For this review, take the finished solid that the model builds, in its own axes (mm). A direction names the side the tool comes from. Give positions to 0.01 mm unless a question says otherwise; leave off trailing zeros. Loops run counter-clockwise (first coordinate to the right, second up) from the corner with the lowest first, then second, coordinate; pieces in that order, holes last. Notation, with made-up numbers: (67, 11) - (94, 11) arc R14 ccw to (94, 35) - close; hole circle Ø8 at (31, -13). An arc over 180 degrees is marked (long way). Answer as CSV lines item,"result".
from build123d import *

# Parameters (mm, degrees)
BASE_FLANGE1_DEPTH = 111.125
SKETCH16_R         = 14.2875
SKETCH16_R_2       = 2.5146
CUT_EXTRUDE1_DEPTH = 191.975656171


# Read off the part's stored shape, not the designer's step: Base-Flange1
with BuildPart() as part:
    # Base-Flange1 outline → Base-Flange1 (new body)
    with BuildSketch(Plane.XY):
        with BuildLine():
            Line((98.425, -3.937), (98.425, -117.475))
            Line((98.425, -117.475), (101.6, -117.475))
            Line((101.6, -117.475), (101.6, -3.937))
            ThreePointArc((101.6, -3.937), (100.446879398, -1.153120602), (97.663, 0))
            Line((97.663, 0), (0, 0))
            Line((0, 0), (0, -3.175))
            Line((0, -3.175), (97.663, -3.175))
            ThreePointArc((97.663, -3.175), (98.201815367, -3.398184633), (98.425, -3.937))
        make_face()
    extrude(amount=BASE_FLANGE1_DEPTH)

    # Sketch16 → Cut-Extrude1 (cut, through all)
    with BuildSketch(Plane(origin=(101.6, 0, 0), x_dir=(0, 0, -1), z_dir=(1, 0, 0))):
        with Locations((-31.75, -84.1375)):
            Circle(SKETCH16_R)
        with Locations((-95.25, -39.6875)):
            Circle(SKETCH16_R)
        with Locations((-38.1, -15.875)):
            Circle(SKETCH16_R_2)
        with Locations((-38.1, -34.925)):
            Circle(SKETCH16_R_2)
        with Locations((-57.15, -15.875)):
            Circle(SKETCH16_R_2)
        with Locations((-57.15, -34.925)):
            Circle(SKETCH16_R_2)
        with Locations((-19.05, -15.875)):
            Circle(SKETCH16_R_2)
        with Locations((-19.05, -34.925)):
            Circle(SKETCH16_R_2)
        Polygon((-58.7375, -117.475), (-111.125, -44.592589994), (-111.125, -117.475), align=None)
    extrude(amount=-CUT_EXTRUDE1_DEPTH, mode=Mode.SUBTRACT)


solid = part.part
1) Wall thickness on line 1 (Y direction, x = 100.35, z = 57.15) (1 decimal); line 2 (X direction, y = -36.5, z = 79.5) (3 decimals); line 3 (Y direction, x = 24, z = 9) (3 decimals): over which ranges is each line inside the solid? List them lowest first. Write a range as from..to.
From the geometry:
line 1,"y = -117.5..-37.4, -32.4..-18.4, -13.4..-1.1"
line 2,"x = 98.425..101.6"
line 3,"y = -3.175..0"
2) Consider section A-A on z = 57.15. Write out the cut boundary in (x, y) (3 decimals), and give its area (3 significant figures).
From the geometry:
outline,"(0, -3.175) - (97.663, -3.175) arc R0.762 cw to (98.425, -3.937) - (98.425, -13.36) - (101.6, -13.36) - (101.6, -3.937) arc R3.937 ccw to (97.663, 0) - (0, 0) - close; (98.425, -117.475) - (101.6, -117.475) - (101.6, -37.44) - (98.425, -37.44) - close; (98.425, -32.41) - (101.6, -32.41) - (101.6, -18.39) - (98.425, -18.39) - close"
area,"650 mm^2"
3) Consider section D-D on z = 38.1. Write out the cut boundary in (x, y) (3 decimals).
From the geometry:
outline,"(0, -3.175) - (97.663, -3.175) arc R0.762 cw to (98.425, -3.937) - (98.425, -13.36) - (101.6, -13.36) - (101.6, -3.937) arc R3.937 ccw to (97.663, 0) - (0, 0) - close; (98.425, -117.475) - (101.6, -117.475) - (101.6, -96.936) - (98.425, -96.936) - close; (98.425, -71.339) - (101.6, -71.339) - (101.6, -37.44) - (98.425, -37.44) - close; (98.425, -32.41) - (101.6, -32.41) - (101.6, -18.39) - (98.425, -18.39) - close"
4) Insertion check: P1, Ø6, axis at y = -15.875, z = 57.15, coming from the -X side (3 decimals); P2, Ø8, axis at x = 46.5, z = 17, coming from the -Y side (3 decimals). Each pin has a flat end and moves straight along its axis. Give the tip position at first contact, or say it passes through.
From the geometry:
P1,"stops at x = 98.425"
P2,"stops at y = -3.175"
5) Consider section B-B on y = -49.5. Write out the cut boundary in (x, z) (3 decimals), and give its area (3 significant figures).
From the geometry:
outline,"(98.425, 0) - (101.6, 0) - (101.6, 84.865) - (98.425, 84.865) - close; (98.425, 105.635) - (101.6, 105.635) - (101.6, 107.598) - (98.425, 107.598) - close"
area,"276 mm^2"
6) Machinability: for faces 1 (the cylindrical face through (100.035, -33.226, 20.903)), 2 (the flat face through (98.425, -47, 42)), which of the approach directions +Z, -Z, +X, -X, +Y, -Y give a long, thin tool a straight path to every point of the face, cutting with its end or side? Answer none if there is none.
From the geometry:
face 1,"+X, -X"
face 2,"+Z, -Z, -X, -Y"
7) Draft analysis for pull direction Z (two halves, no side actions). For faces 3 (the cylindrical face through (100.03, -34.17, 54.75)), 4 (the flat face through (66, -2, 111.125)), 5 (the cylindrical face through (100.03, -15.12, 54.75)), 6 (the flat face through (101.6, -49, 42)), state which applies: pulls with the +Z half, pulls with the -Z half, needs draft (parallel to the pull), parting line crosses it, or undercut.
From the geometry:
face 3,"undercut"
face 4,"pulls with the +Z half"
face 5,"undercut"
face 6,"needs draft"
8) Consider section C-C on z = 95.25. Write out the cut boundary in (x, y) (3 decimals), and give its area (3 significant figures).
From the geometry:
outline,"(0, -3.175) - (97.663, -3.175) arc R0.762 cw to (98.425, -3.937) - (98.425, -25.4) - (101.6, -25.4) - (101.6, -3.937) arc R3.937 ccw to (97.663, 0) - (0, 0) - close; (98.425, -66.678) - (101.6, -66.678) - (101.6, -53.975) - (98.425, -53.975) - close"
area,"430 mm^2"
